```python
from build123d import *

# Parameters (mm, degrees)
F0_W     = 15.7
F0_H     = 7.7
F0_W_2   = 12.5
F0_H_2   = 4.5
F1_DEPTH = 1.5
F2_DEPTH = 14.3
F3_W     = 2.2
F3_H     = 1.25
F4_DEPTH = 0.2


with BuildPart() as f1:
    # F0 (on Top) → F1 (new body)
    with BuildSketch(Plane.XY):
        Rectangle(F0_W, F0_H)
        Rectangle(F0_W_2, F0_H_2, mode=Mode.SUBTRACT)
        Rectangle(F0_W_2, F0_H_2)
    extrude(amount=F1_DEPTH)

    # F0 (on Top) → F2 (join)
    with BuildSketch(Plane.XY):
        Rectangle(F0_W, F0_H)
        Rectangle(F0_W_2, F0_H_2, mode=Mode.SUBTRACT)
    extrude(amount=F2_DEPTH)

    # F3 (on face) → F4 (join)
    with BuildSketch(Plane.XZ.offset(-2.25)):
        with Locations((3.65, 8.175)):
            Rectangle(F3_W, F3_H)
        with Locations((-3.65, 8.175)):
            Rectangle(F3_W, F3_H)
    extrude(amount=F4_DEPTH)


solid = f1.part
```
Geometry: final body of the model. Coordinates: model frame, mm. A direction names the side the tool comes from. Round coordinates to 2 decimals unless told otherwise and drop trailing zeros. Order: outer loops, then holes, each group sorted by start corner. A loop starts at its lowest first (then second) coordinate and runs counter-clockwise, first axis right, second up. Notation, with made-up numbers: (-16, 83.25) - (0, 83.25) arc R20 cw to (0, 92.25) - close; hole circle Ø8 at (-19.5, 56). An arc over 180 degrees is marked (long way). Write item = value, one per line. Start each with the question number.
Q1. Ray query, line 1 (Y direction, x = 2, z = 8.25); line 2 (X direction, y = -2, z = 7.5); line 3 (Z direction, x = -1.25, y = 1.5). Return the intervals inside material, ascending. Write a range as from..to.
Q2. Pin query (flat end, axial travel): pin 1 (2 mm diameter, centred on x = -0.5, y = 0.5, fed in from +Z). Return the tip coordinate at first contact, or that it passes through.
Q3. Access query for faces 1 (the flat face through (0, 0, 0)), 2 (the flat face through (-6.25, 0, 8)), 3 (the flat face through (0, 2.25, 8)). Directions: +Z, -Z, +X, -X, +Y, -Y. A direction counts if a zero-diameter tool reaches every point of the face in a straight line with its end or side. Return the directions, or none.
Q4. Pull-direction query (Y, two-part tool) for faces 4 (the flat face through (0, -3.85, 7)), 5 (the flat face through (-4, 2.05, 8)), 6 (the flat face through (7.85, 0, 7)); classes: +Y half, -Y half, draft (parallel to the pull), parting line (faces both ways), or undercut.
Q5. Cut plane A-A on z = 13.25. Return the cut outline in (x, y).
Q6. Cut plane C-C on y = -2. Return the cut outline in (x, z).
Q7. Cut plane B-B on x = -5. Return the cut outline in (y, z).
Outcome:
q1.line_1 = -3.85..-2.25, 2.25..3.85
q1.line_2 = -7.85..-6.25, 6.25..7.85
q1.line_3 = 0..1.5
q2.pin_1 = 1.5
q3.face_1 = -Z, +X, -X, +Y, -Y
q3.face_2 = +Z
q3.face_3 = none
q4.face_4 = -Y half
q4.face_5 = undercut
q4.face_6 = draft
q5.outline = (-7.85, -3.85) - (7.85, -3.85) - (7.85, 3.85) - (-7.85, 3.85) - close; hole (-6.25, -2.25) - (6.25, -2.25) - (6.25, 2.25) - (-6.25, 2.25) - close
q6.outline = (-7.85, 0) - (7.85, 0) - (7.85, 14.3) - (6.25, 14.3) - (6.25, 1.5) - (-6.25, 1.5) - (-6.25, 14.3) - (-7.85, 14.3) - close
q7.outline = (-3.85, 0) - (3.85, 0) - (3.85, 14.3) - (2.25, 14.3) - (2.25, 1.5) - (-2.25, 1.5) - (-2.25, 14.3) - (-3.85, 14.3) - close
